CAD build for the part. Positions are in the model's coordinates, mm. Face numbers are marked on the shaded views. A direction names the side the tool comes from. Round coordinates to 2 decimals unless told otherwise and drop trailing zeros. Loops run counter-clockwise (first coordinate to the right, second up) from the corner with the lowest first, then second, coordinate; pieces in that order, holes last. Notation, with made-up numbers: M 0.25,15 L 18.25,15 A20 cw 18.25,42 Z; hole C 4.5,31.5 d1. An arc over 180 degrees is marked long. One line per item, written item: value. Start each with the question number.
from build123d import *

# Parameters (mm, degrees)
SKETCH2_R               = 0.35
BOSS_EXTRUDE2_DEPTH     = 10
SKETCH4_R               = 3.5
BOSS_EXTRUDE3_DEPTH     = 10
CHAMFER1_SIZE           = 3.05
CHAMFER1_SIZE2          = 5.282754963
CUT_EXTRUDE4_DEPTH      = 21.603397778
CUT_EXTRUDE4_DEPTH_BACK = 21.603397778
SKETCH5_R               = 1
SKETCH6_R               = 1.5
BOSS_EXTRUDE4_DEPTH     = 1
SKETCH7_R               = 2
BOSS_EXTRUDE5_DEPTH     = 4
CHAMFER2_SIZE           = 0.5


with BuildPart() as part:
    # Sketch1 → Revolve1 (revolve)
    with BuildSketch(Plane.XY):
        with BuildLine():
            Line((0, 0), (0, -1))
            ThreePointArc((0, -1), (1, 0), (0, 1))
            Line((0, 1), (0, 0))
        make_face()
    revolve(axis=Axis((0, 0, 0), (0, 1, 0)))

    # Sketch2 → Boss-Extrude2 (add)
    with BuildSketch(Plane(origin=(0, 0, 0), x_dir=(1, 0, 0), z_dir=(0, 1, 0))):
        with Locations(Location((0, 0, 0), (0, 0, 90))):
            Circle(SKETCH2_R)
    extrude(amount=BOSS_EXTRUDE2_DEPTH)

    # Sketch4 → Boss-Extrude3 (add)
    with BuildSketch(Plane(origin=(0, 10, 0), x_dir=(1, 0, 0), z_dir=(0, 1, 0))):
        with Locations(Location((0, 0, 0), (0, 0, 270))):
            Circle(SKETCH4_R)
    extrude(amount=BOSS_EXTRUDE3_DEPTH)

    # Chamfer1
    chamfer1_edges = [part.edges().sort_by_distance(p)[0] for p in [
        (0, 10, -3.5),
    ]]
    chamfer1_side = [part.faces().sort_by_distance(p)[0] for p in [
        (0, 10, -3.401005051),
    ]]
    chamfer(chamfer1_edges, length=CHAMFER1_SIZE, length2=CHAMFER1_SIZE2, reference=chamfer1_side[0])

    # Sketch5 → Cut-Extrude4 (cut, two sides: drawn at the far end of the back side and taken through both)
    with BuildSketch(Plane(origin=(0, 0, 0), x_dir=(0, 0, -1), z_dir=(1, 0, 0)).offset(-CUT_EXTRUDE4_DEPTH_BACK)):
        with Locations((0, 17.641377482)):
            Circle(SKETCH5_R)
    extrude(amount=CUT_EXTRUDE4_DEPTH + CUT_EXTRUDE4_DEPTH_BACK, mode=Mode.SUBTRACT)

    # Sketch6 → Boss-Extrude4 (add)
    with BuildSketch(Plane(origin=(0, 20, 0), x_dir=(1, 0, 0), z_dir=(0, 1, 0))):
        with Locations(Location((0, 0, 0), (0, 0, 270))):
            Circle(SKETCH6_R)
    extrude(amount=BOSS_EXTRUDE4_DEPTH)

    # Sketch7 → Boss-Extrude5 (add)
    with BuildSketch(Plane(origin=(0, 21, 0), x_dir=(1, 0, 0), z_dir=(0, 1, 0))):
        with Locations(Location((0, 0, 0), (0, 0, 270))):
            Circle(SKETCH7_R)
    extrude(amount=BOSS_EXTRUDE5_DEPTH)

    # Chamfer2
    chamfer2_edges = [part.edges().sort_by_distance(p)[0] for p in [
        (0, 21, -2),
        (0, 25, -2),
    ]]
    chamfer(chamfer2_edges, length=CHAMFER2_SIZE - 0.0001)  # a hair under: the kernel refuses the full size


solid = part.part
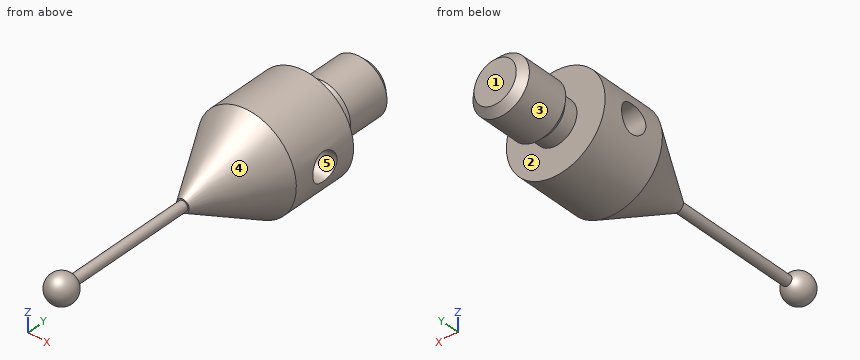
(1) Probe L1, parallel to Y at x = 1.75, z = 0; L2, parallel to Y at x = 0.5, z = 0; L3, parallel to Y at x = -2, z = 0.5. List the from-to ranges inside material, lowest first.
(2) Mould opens along Y. For the marked faces 1, 2 and 3 say: pulls with the +Y half, pulls with the -Y half, needs draft (parallel to the pull), parting line crosses it, or undercut.
(3) Which spindle directions (+Z, -Z, +X, -X, +Y, -Y) get a long thin tool onto all of the face, cutting with end or side? Do the marked faces 4 and 5. Say none if no direction does.
(4) Slice it at C-C, the plane y = 10.75. List the corners of the cut face in (x, z).
(5) Slice it at D-D, the plane y = 13.75. List the corners of the cut face in (x, z), and give its area (3 significant figures).
(6) Flat gauge pin, fed straight in: P1, Ø4, axis at x = 2, z = -1.5, coming from the -Y side. Where does the tip first touch, or does it go through?
Check result:
1. L1: y = 12.25 to 16.64, 18.64 to 20, 21.25 to 24.75
1. L2: y = -0.87 to 0.87, 10.09 to 16.64, 18.64 to 25
1. L3: y = 12.79 to 16.78, 18.51 to 20
2. face 1: pulls with the +Y half
2. face 2: undercut
2. face 3: needs draft
3. face 4: none
3. face 5: +X, -X
4. outline: C 0,0 d1.77
5. outline: C 0,0 d5.23
5. area: 21.5 mm^2
6. P1: stops at y = -0.87
